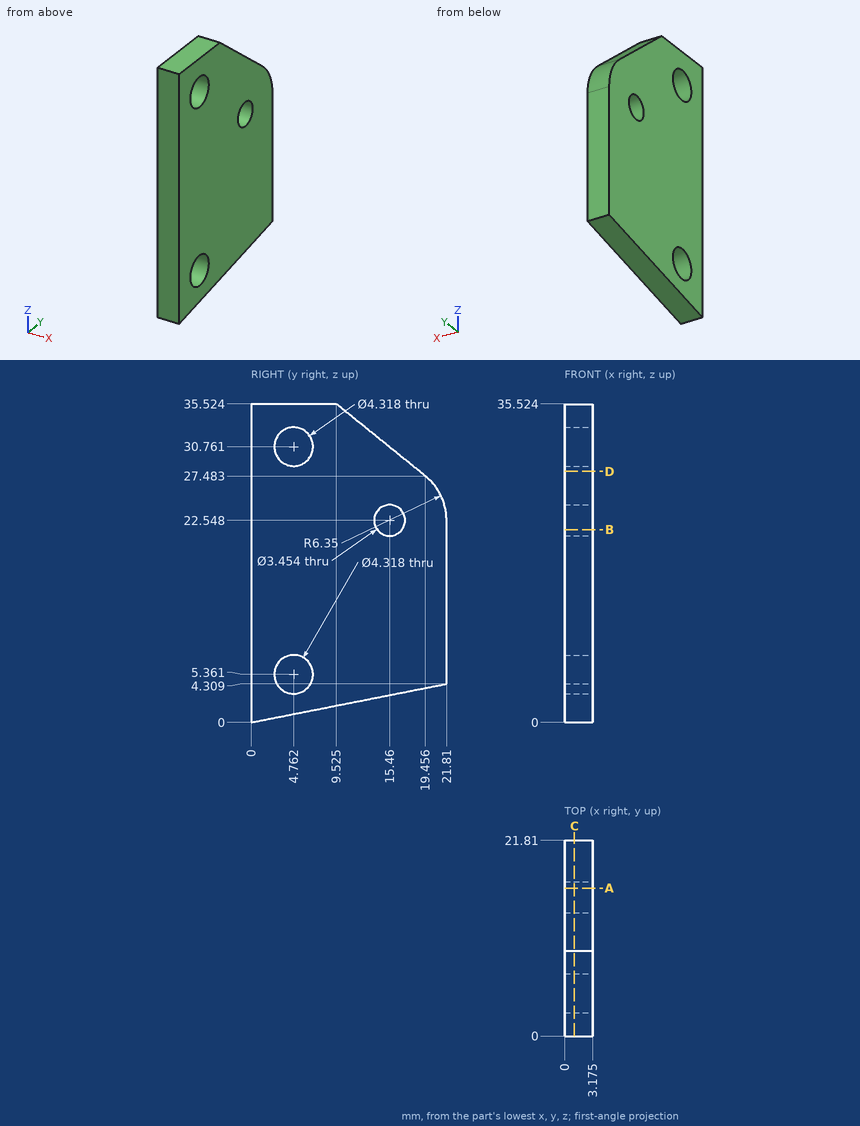
Part print with two shaded views. Sizes in mm from the minimum x, y, z corner. Give positions to 0.01 mm unless a question says otherwise; leave off trailing zeros. Write each loop counter-clockwise with the first axis right and the second up, starting at its lowest first coordinate (ties: lowest second). Pieces come first, ordered by that corner, then holes.
1) Pin check, flat tip, straight feed: pin 1 (5 mm diameter, centred on y = 4.76, z = 5.36, fed in from -X). Stop position of the tip, or through.
Resolved:
pin 1: stops at x = 0
2) Cut at D-D on z = 28. Write the cut outline in (x, y) (1 decimal).
Resolved:
outline: (0, 0) - (3.2, 0) - (3.2, 18.8) - (0, 18.8) - close
3) Cut at A-A on y = 16.5. Write the cut outline in (x, z) (1 decimal).
Resolved:
outline: (0, 3.3) - (3.2, 3.3) - (3.2, 21.2) - (0, 21.2) - close; (0, 23.9) - (3.2, 23.9) - (3.2, 29.9) - (0, 29.9) - close
4) Cut at C-C on x = 1.1. State how many separate pieces and enclosed holes the cut face has, then the cut area to 3 significant figures.
Resolved:
separate pieces: 1
enclosed holes: 3
area: 627 mm2
5) Cut at B-B on z = 21.5. Write the cut outline in (x, y) (1 decimal).
Resolved:
outline: (0, 0) - (3.2, 0) - (3.2, 14.1) - (0, 14.1) - close; (0, 16.8) - (3.2, 16.8) - (3.2, 21.8) - (0, 21.8) - close
6) Probe L1, parallel to Z at x = 0.8, y = 3.25 (1 decimal); L2, parallel to Z at x = 1.7, y = 15.25 (1 decimal); L3, parallel to Y at x = 1.9, z = 32 (1 decimal). List the from-to ranges inside material, lowest first.
Resolved:
L1: z = 0.6 to 3.8, 6.9 to 29.2, 32.3 to 35.5
L2: z = 3 to 20.8, 24.3 to 30.9
L3: y = 0 to 3, 6.5 to 13.9
